Work out the finished part from the listing and answer in its coordinate system (mm). Face numbers are marked on the shaded views. A direction names the side the tool comes from. Round coordinates to 2 decimals unless told otherwise and drop trailing zeros. Order: outer loops, then holes, each group sorted by start corner. A loop starts at its lowest first (then second) coordinate and runs counter-clockwise, first axis right, second up. Notation, with made-up numbers: (87.25, 68) -> (95.25, 68) arc R9 cw to (95.25, 83) -> close; hole circle Ø7 at (26.5, 0.25). An arc over 180 degrees is marked (long way). Use a Markdown table: item, result. Add a question column.
Item 1: Flat-ended cylindrical pins translate along their axes: P1, Ø2, axis at y = 19.5, z = 11.5, coming from the +X side; P2, Ø10, axis at x = -42.5, z = 9.5, coming from the -Y side; P3, Ø12, axis at x = 2, y = 3, coming from the -Z side; P4, Ø10, axis at x = -45, y = 14, coming from the -Z side. Find the tip coordinate at first contact, or state that the pin passes through.
Item 2: Find the intervals of material crossed by L1, parallel to X at y = 0, z = 6.2; L2, parallel to X at y = 12, z = 6.5; L3, parallel to Y at x = 0, z = 2.8, in increasing order. Write a range as [from, to].
Item 3: A cutting plane is placed at A-A, the plane x = 0. Determine the outline of the cut face in (y, z).
Item 4: For a pull along Y with two mould halves and no side action, classify the marked faces 1 and 2 as +Y half, -Y half, draft (parallel to the pull), parting line (faces both ways), or undercut.
Item 5: A tool of negligible diameter and unlimited length cuts with its end or side. For the marked faces 3, 4 and 5, from which of +Z, -Z, +X, -X, +Y, -Y can it reach the whole face along a straight path? Write none if from no direction.
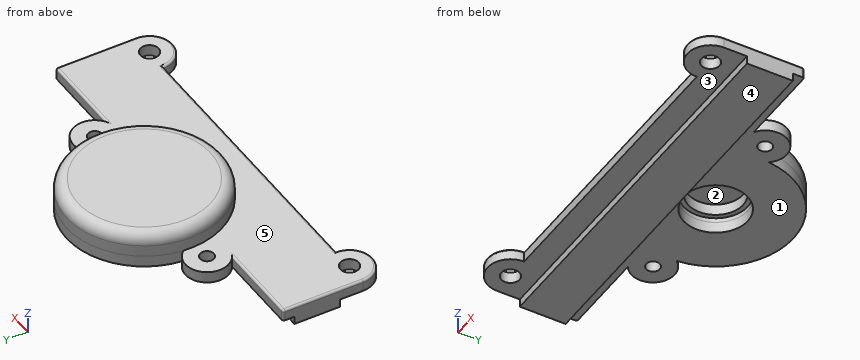
from build123d import *

# Parameters (mm, degrees)
SKETCH1_R           = 4
SKETCH1_R_2         = 3
SKETCH1_R_3         = 14
BOSS_EXTRUDE2_DEPTH = 5
SKETCH2_R           = 33.920814748
BOSS_EXTRUDE3_DEPTH = 10
BOSS_EXTRUDE4_DEPTH = 3.5
SKETCH5_R           = 14
CUT_EXTRUDE1_DEPTH  = 2
FILLET1_R           = 5
SKETCH6_R           = 12
CUT_EXTRUDE2_DEPTH  = 5
FILLET2_R           = 1


with BuildPart() as part:
    # Sketch1 → Boss-Extrude2 (new body)
    with BuildSketch(Plane.XY):
        with BuildLine():
            Line((-83.333333333, -10.859226218), (-83.333333333, -35.859226218))
            Line((-83.333333333, -35.859226218), (-83.333333333, -45.859226218))
            ThreePointArc((-83.333333333, -45.859226218), (-73.333333333, -55.859226218), (-63.333333333, -45.859226218))
            Line((-63.333333333, -45.859226218), (0, -45.859226218))
            Line((0, -45.859226218), (63.333333333, -45.859226218))
            ThreePointArc((63.333333333, -45.859226218), (73.333333333, -55.859226218), (83.333333333, -45.859226218))
            Line((83.333333333, -45.859226218), (83.333333333, -35.859226218))
            Line((83.333333333, -35.859226218), (83.333333333, -10.859226218))
            Line((83.333333333, -10.859226218), (46.135632545, -10.859226218))
            ThreePointArc((46.135632545, -10.859226218), (48.189979587, 3.404653395), (33.783237398, 3.051973795))
            ThreePointArc((33.783237398, 3.051973795), (0, 33.920814748), (-33.783237398, 3.051973795))
            ThreePointArc((-33.783237398, 3.051973795), (-48.189979587, 3.404653395), (-46.135632545, -10.859226218))
            Line((-46.135632545, -10.859226218), (-83.333333333, -10.859226218))
        make_face()
        with Locations((-73.333333333, -45.859226218)):
            Circle(SKETCH1_R, mode=Mode.SUBTRACT)
        with Locations((73.333333333, -45.859226218)):
            Circle(SKETCH1_R, mode=Mode.SUBTRACT)
        with Locations((-41.135632545, -2.859226218)):
            Circle(SKETCH1_R_2, mode=Mode.SUBTRACT)
        Circle(SKETCH1_R_3, mode=Mode.SUBTRACT)
        with Locations((41.135632545, -2.859226218)):
            Circle(SKETCH1_R_2, mode=Mode.SUBTRACT)
    extrude(amount=BOSS_EXTRUDE2_DEPTH)

    # Sketch2 → Boss-Extrude3 (add)
    with BuildSketch(Plane.XY.offset(5)):
        with Locations(Location((0, 0, 0), (0, 0, 174.837918502))):
            Circle(SKETCH2_R)
    extrude(amount=BOSS_EXTRUDE3_DEPTH)

    # Sketch3 → Boss-Extrude4 (add)
    with BuildSketch(Plane(origin=(0, 0, 0), x_dir=(-1, 0, 0), z_dir=(0, 0, -1))):
        Polygon((-83.333333333, -35.859226218), (83.333333333, -35.859226218), (83.333333333, -15.859226218), (-5.229680356, -15.859226218), (-83.333333333, -15.859226218), align=None)
    extrude(amount=BOSS_EXTRUDE4_DEPTH)

    # Sketch5 → Cut-Extrude1 (cut)
    with BuildSketch(Plane(origin=(0, 0, 5), x_dir=(-1, 0, 0), z_dir=(0, 0, -1))):
        Circle(SKETCH5_R)
    extrude(amount=-CUT_EXTRUDE1_DEPTH, mode=Mode.SUBTRACT)

    # Fillet1
    fillet1_edges = [part.edges().sort_by_distance(p)[0] for p in [
        (33.783237398, -3.051973795, 15),
    ]]
    fillet(fillet1_edges, radius=FILLET1_R)

    # Sketch6 → Cut-Extrude2 (cut)
    with BuildSketch(Plane(origin=(0, 0, 7), x_dir=(-1, 0, 0), z_dir=(0, 0, -1))):
        Circle(SKETCH6_R)
    extrude(amount=-CUT_EXTRUDE2_DEPTH, mode=Mode.SUBTRACT)

    # Fillet2
    fillet2_edges = [part.edges().sort_by_distance(p)[0] for p in [
        (83.333333333, -10.859226218, 2.5),
        (-83.333333333, -10.859226218, 2.5),
        (64.734482939, -10.859226218, 5),
        (-64.734482939, -10.859226218, 5),
        (-83.333333333, -28.359226218, 5),
        (-73.333333333, -55.859226218, 5),
        (0, -45.859226218, 5),
        (73.333333333, -55.859226218, 5),
        (83.333333333, -28.359226218, 5),
    ]]
    fillet(fillet2_edges, radius=FILLET2_R)


solid = part.part
Reported:
| question | item | result |
|---|---|---|
| 1 | P1 | x = 28.23 |
| 1 | P2 | y = -45.73 |
| 1 | P3 | z = 12 |
| 1 | P4 | through |
| 2 | L1 | [-33.92, -14], [14, 33.92] |
| 2 | L2 | [-31.73, -7.21], [7.21, 31.73] |
| 2 | L3 | [-45.86, -14], [14, 33.92] |
| 3 | outline | (-45.86, 0) -> (-35.86, 0) -> (-35.86, -3.5) -> (-15.86, -3.5) -> (-15.86, 0) -> (-14, 0) -> (-14, 7) -> (-12, 7) -> (-12, 12) -> (12, 12) -> (12, 7) -> (14, 7) -> (14, 0) -> (33.92, 0) -> (33.92, 10) arc R5 ccw to (28.92, 15) -> (-28.92, 15) arc R5 ccw to (-33.92, 10) -> (-33.92, 5) -> (-44.86, 5) arc R1 ccw to (-45.86, 4) -> close |
| 4 | face 1 | draft |
| 4 | face 2 | undercut |
| 5 | face 3 | -Z, +X, -X, -Y |
| 5 | face 4 | -Z, +X, -X, +Y, -Y |
| 5 | face 5 | +Z, -Y |
